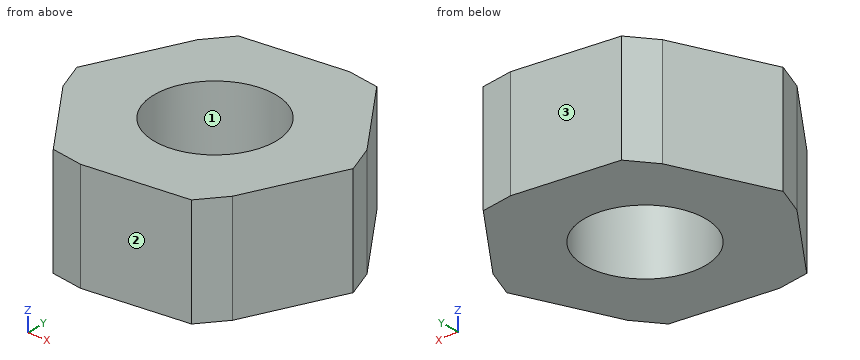
from build123d import *
from OCP.BRepFilletAPI import BRepFilletAPI_MakeChamfer

# Parameters (mm, degrees)
RESSALTO_EXTRUS_O1_DEPTH = 4.5
ESBO_O2_R                = 2.5
CORTE_EXTRUS_O1_DEPTH    = 7.5
CHANFRO1_SIZE            = 0.4
CHANFRO1_SIZE2           = 1.092820323


with BuildPart() as part:
    # Esboço1 → Ressalto-extrusão1 (new body)
    with BuildSketch(Plane.XY):
        Polygon((-5.144411163, -2.872547916), (-2.753633945, 2.382689246), (-6.109414221, 7.080781632), (-11.855971715, 6.523636857), (-14.246748933, 1.268399695), (-10.890968657, -3.429692692), align=None)
    extrude(amount=RESSALTO_EXTRUS_O1_DEPTH)

    # Esboço2 → Corte-extrusão1 (cut)
    with BuildSketch(Plane.XY.offset(4.5)):
        with Locations((-8.500191439, 1.82554447)):
            Circle(ESBO_O2_R)
    extrude(amount=-CORTE_EXTRUS_O1_DEPTH, mode=Mode.SUBTRACT)

    # Chanfro1: one chamfer whose edges measure the first distance from different faces: ONE call of the kernel's chamfer builder (chamfer() names one face for all edges)
    chanfro1_edges_1 = [part.edges().sort_by_distance(p)[0] for p in [
        (-10.890968657, -3.429692692, 2.25),
    ]]
    chanfro1_side_1 = [part.faces().sort_by_distance(p)[0] for p in [
        (-12.568858795, -1.080646498, 2.25),
    ]]
    chanfro1_edges_2 = [part.edges().sort_by_distance(p)[0] for p in [
        (-14.246748933, 1.268399695, 2.25),
    ]]
    chanfro1_side_2 = [part.faces().sort_by_distance(p)[0] for p in [
        (-13.051360324, 3.896018276, 2.25),
    ]]
    chanfro1_edges_3 = [part.edges().sort_by_distance(p)[0] for p in [
        (-11.855971715, 6.523636857, 2.25),
    ]]
    chanfro1_side_3 = [part.faces().sort_by_distance(p)[0] for p in [
        (-8.982692968, 6.802209244, 2.25),
    ]]
    chanfro1_edges_4 = [part.edges().sort_by_distance(p)[0] for p in [
        (-6.109414221, 7.080781632, 2.25),
    ]]
    chanfro1_side_4 = [part.faces().sort_by_distance(p)[0] for p in [
        (-4.431524083, 4.731735439, 2.25),
    ]]
    chanfro1_edges_5 = [part.edges().sort_by_distance(p)[0] for p in [
        (-2.753633945, 2.382689246, 2.25),
    ]]
    chanfro1_side_5 = [part.faces().sort_by_distance(p)[0] for p in [
        (-3.949022554, -0.244929335, 2.25),
    ]]
    chanfro1_edges_6 = [part.edges().sort_by_distance(p)[0] for p in [
        (-5.144411163, -2.872547916, 2.25),
    ]]
    chanfro1_side_6 = [part.faces().sort_by_distance(p)[0] for p in [
        (-8.01768991, -3.151120304, 2.25),
    ]]
    chanfro1 = BRepFilletAPI_MakeChamfer(part.part.solid().wrapped)
    for e in chanfro1_edges_1:
        chanfro1.Add(CHANFRO1_SIZE, CHANFRO1_SIZE2, e.wrapped, chanfro1_side_1[0].wrapped)  # the first distance lies on this face
    for e in chanfro1_edges_2:
        chanfro1.Add(CHANFRO1_SIZE, CHANFRO1_SIZE2, e.wrapped, chanfro1_side_2[0].wrapped)  # the first distance lies on this face
    for e in chanfro1_edges_3:
        chanfro1.Add(CHANFRO1_SIZE, CHANFRO1_SIZE2, e.wrapped, chanfro1_side_3[0].wrapped)  # the first distance lies on this face
    for e in chanfro1_edges_4:
        chanfro1.Add(CHANFRO1_SIZE, CHANFRO1_SIZE2, e.wrapped, chanfro1_side_4[0].wrapped)  # the first distance lies on this face
    for e in chanfro1_edges_5:
        chanfro1.Add(CHANFRO1_SIZE, CHANFRO1_SIZE2, e.wrapped, chanfro1_side_5[0].wrapped)  # the first distance lies on this face
    for e in chanfro1_edges_6:
        chanfro1.Add(CHANFRO1_SIZE, CHANFRO1_SIZE2, e.wrapped, chanfro1_side_6[0].wrapped)  # the first distance lies on this face
    add(Compound.cast(chanfro1.Shape()), mode=Mode.REPLACE)


solid = part.part
Model file for the job. Use its own axes, mm. Face numbers are marked on the shaded views. Give positions to 0.01 mm unless a question says otherwise; leave off trailing zeros. Write each loop counter-clockwise with the first axis right and the second up, starting at its lowest first coordinate (ties: lowest second). Pieces come first, ordered by that corner, then holes. Notation, with made-up numbers: (44.25, 85) -> (57.25, 85) arc R18 cw to (57.25, 118) -> close; hole circle Ø6 at (61.25, 53). An arc over 180 degrees is marked (long way). Write item = value, one per line.
(1) Slice it at D-D, the plane x = -3.25. Give the cut face in (y, z), then the cut area to 3 significant figures.
Determined:
outline = (1.29, 0) -> (2.9, 0) -> (2.9, 4.5) -> (1.29, 4.5) -> close
area = 7.24 mm2
(2) Mould opens along X. For the marked faces 1, 2 and 3 say: released by +X, released by -X, zero draft, split by the parting line, or undercut.
Determined:
face_1 = undercut
face_2 = released by +X
face_3 = released by -X
(3) Probe line 1 along X through (y, z) = (2, 1.7); line 2 along Y through (x, z) = (-6.25, 2.05); line 3 along X through (y, z) = (3.25, 2.9). List the from-to ranges inside material, lowest first.
Determined:
line_1 = -13.91 to -10.99, -6.01 to -2.93
line_2 = -2.98 to 0.74, 2.91 to 6.82
line_3 = -13.35 to -10.55, -6.45 to -3.38
(4) Flat gauge pins, fed straight in: P1, Ø1, axis at x = -7.5, y = 1, coming from the -Z side; P2, Ø2, axis at y = -2, z = 2, coming from the -X side. Where does each tip first touch, or does it go through?
Determined:
P1 = through
P2 = -12.63
(5) Slice it at A-A, the plane y = 4. Give the cut face in (x, z), then the cut area to 3 significant figures.
Determined:
outline = (-13, 0) -> (-9.73, 0) -> (-9.73, 4.5) -> (-13, 4.5) -> close; (-7.27, 0) -> (-3.91, 0) -> (-3.91, 4.5) -> (-7.27, 4.5) -> close
area = 29.8 mm2
(6) Slice it at B-B, the plane z = 2.8. Give the cut face in (x, y).
Determined:
outline = (-14.08, 1.63) -> (-13.61, 0.38) -> (-11.12, -3.1) -> (-9.8, -3.32) -> (-5.54, -2.91) -> (-4.69, -1.88) -> (-2.92, 2.02) -> (-3.39, 3.27) -> (-5.88, 6.76) -> (-7.2, 6.98) -> (-11.46, 6.56) -> (-12.31, 5.53) -> close; hole circle Ø5 at (-8.5, 1.83)
(7) Slice it at C-C, the plane x = -8.5. Give the cut face in (y, z).
Determined:
outline = (-3.2, 0) -> (-0.67, 0) -> (-0.67, 4.5) -> (-3.2, 4.5) -> close; (4.33, 0) -> (6.85, 0) -> (6.85, 4.5) -> (4.33, 4.5) -> close
